```python
from build123d import *

# Parameters (mm, degrees)
F1_DEPTH = 50
F2_DEPTH = 25


with BuildPart() as f1:
    # F0 (on Front) → F1 (new body)
    with BuildSketch(Plane.XZ):
        with BuildLine():
            ThreePointArc((60.3004275437, 340.9588258691), (82.833452945, 336.1958976151), (105, 329.9455447494))
            Line((105, 329.9455447494), (105, 360))
            ThreePointArc((105, 360), (0, 375), (-105, 360))
            Line((-105, 360), (-105, 329.9455447494))
            ThreePointArc((-105, 329.9455447494), (-82.833452945, 336.1958976151), (-60.3004275437, 340.9588258691))
            ThreePointArc((-60.3004275437, 340.9588258691), (-44.7093862816, 361.4956891559), (-24.5847162741, 345.3761054643))
            ThreePointArc((-24.5847162741, 345.3761054643), (-17.7950983093, 345.7924189108), (-10.9986121712, 346.0752707581))
            ThreePointArc((-10.9986121712, 346.0752707581), (-0.0873673767, 357.2496530373), (11, 346.25))
            ThreePointArc((11, 346.25), (10.9996530373, 346.1626326233), (10.9986121712, 346.0752707581))
            ThreePointArc((10.9986121712, 346.0752707581), (17.7950983093, 345.7924189108), (24.5847162741, 345.3761054643))
            ThreePointArc((24.5847162741, 345.3761054643), (43.3731818064, 361.6106063163), (60.5, 343.6317978593))
            ThreePointArc((60.5, 343.6317978593), (60.4500375457, 342.2915918653), (60.3004275437, 340.9588258691))
        make_face()
        with BuildLine():
            ThreePointArc((-105, 299.635194862), (0, 317.5), (105, 299.635194862))
            Line((105, 299.635194862), (105, 329.9455447494))
            ThreePointArc((105, 329.9455447494), (82.833452945, 336.1958976151), (60.3004275437, 340.9588258691))
            ThreePointArc((60.3004275437, 340.9588258691), (40.2906137184, 325.7679065626), (24.5847162741, 345.3761054643))
            ThreePointArc((24.5847162741, 345.3761054643), (17.7950983093, 345.7924189108), (10.9986121712, 346.0752707581))
            ThreePointArc((10.9986121712, 346.0752707581), (0, 335.25), (-10.9986121712, 346.0752707581))
            ThreePointArc((-10.9986121712, 346.0752707581), (-17.7950983093, 345.7924189108), (-24.5847162741, 345.3761054643))
            ThreePointArc((-24.5847162741, 345.3761054643), (-24.521191543, 344.5049796657), (-24.5, 343.6317978593))
            ThreePointArc((-24.5, 343.6317978593), (-41.159794006, 325.6817603135), (-60.3004275437, 340.9588258691))
            ThreePointArc((-60.3004275437, 340.9588258691), (-82.833452945, 336.1958976151), (-105, 329.9455447494))
            Line((-105, 329.9455447494), (-105, 299.635194862))
        make_face()
        with BuildLine():
            ThreePointArc((-24.5847162741, 345.3761054643), (-44.7093862816, 361.4956891559), (-60.3004275437, 340.9588258691))
            ThreePointArc((-60.3004275437, 340.9588258691), (-57.8364575566, 341.3854224733), (-55.3694709553, 341.7942132133))
            ThreePointArc((-55.3694709553, 341.7942132133), (-44.09566787, 356.5334971291), (-29.5706194929, 344.9849865759))
            ThreePointArc((-29.5706194929, 344.9849865759), (-27.0783740558, 345.1895481594), (-24.5847162741, 345.3761054643))
        make_face()
        with BuildLine():
            ThreePointArc((-55.3694709553, 341.7942132133), (-57.8364575566, 341.3854224733), (-60.3004275437, 340.9588258691))
            ThreePointArc((-60.3004275437, 340.9588258691), (-41.159794006, 325.6817603135), (-24.5, 343.6317978593))
            ThreePointArc((-24.5, 343.6317978593), (-24.521191543, 344.5049796657), (-24.5847162741, 345.3761054643))
            ThreePointArc((-24.5847162741, 345.3761054643), (-27.0783740558, 345.1895481594), (-29.5706194929, 344.9849865759))
            ThreePointArc((-29.5706194929, 344.9849865759), (-29.5176668778, 344.3093129543), (-29.5, 343.6317978593))
            ThreePointArc((-29.5, 343.6317978593), (-41.5788926281, 330.6644711799), (-55.3694709553, 341.7942132133))
        make_face()
        with BuildLine():
            ThreePointArc((55.3694709553, 341.7942132133), (57.8364575566, 341.3854224733), (60.3004275437, 340.9588258691))
            ThreePointArc((60.3004275437, 340.9588258691), (60.4500375457, 342.2915918653), (60.5, 343.6317978593))
            ThreePointArc((60.5, 343.6317978593), (43.3731818064, 361.6106063163), (24.5847162741, 345.3761054643))
            ThreePointArc((24.5847162741, 345.3761054643), (27.0783740558, 345.1895481594), (29.5706194929, 344.9849865759))
            ThreePointArc((29.5706194929, 344.9849865759), (43.177515095, 356.6141309815), (55.5, 343.6317978593))
            ThreePointArc((55.5, 343.6317978593), (55.4673266794, 342.7106904874), (55.3694709553, 341.7942132133))
        make_face()
        with BuildLine():
            ThreePointArc((24.5847162741, 345.3761054643), (40.2906137184, 325.7679065626), (60.3004275437, 340.9588258691))
            ThreePointArc((60.3004275437, 340.9588258691), (57.8364575566, 341.3854224733), (55.3694709553, 341.7942132133))
            ThreePointArc((55.3694709553, 341.7942132133), (40.90433213, 330.7300985895), (29.5706194929, 344.9849865759))
            ThreePointArc((29.5706194929, 344.9849865759), (27.0783740558, 345.1895481594), (24.5847162741, 345.3761054643))
        make_face()
    extrude(amount=-F1_DEPTH)

    # F0 (on Front) → F2 (cut)
    with BuildSketch(Plane.XZ):
        with BuildLine():
            ThreePointArc((-24.5847162741, 345.3761054643), (-44.7093862816, 361.4956891559), (-60.3004275437, 340.9588258691))
            ThreePointArc((-60.3004275437, 340.9588258691), (-57.8364575566, 341.3854224733), (-55.3694709553, 341.7942132133))
            ThreePointArc((-55.3694709553, 341.7942132133), (-44.09566787, 356.5334971291), (-29.5706194929, 344.9849865759))
            ThreePointArc((-29.5706194929, 344.9849865759), (-27.0783740558, 345.1895481594), (-24.5847162741, 345.3761054643))
        make_face()
        with BuildLine():
            ThreePointArc((-55.3694709553, 341.7942132133), (-57.8364575566, 341.3854224733), (-60.3004275437, 340.9588258691))
            ThreePointArc((-60.3004275437, 340.9588258691), (-41.159794006, 325.6817603135), (-24.5, 343.6317978593))
            ThreePointArc((-24.5, 343.6317978593), (-24.521191543, 344.5049796657), (-24.5847162741, 345.3761054643))
            ThreePointArc((-24.5847162741, 345.3761054643), (-27.0783740558, 345.1895481594), (-29.5706194929, 344.9849865759))
            ThreePointArc((-29.5706194929, 344.9849865759), (-29.5176668778, 344.3093129543), (-29.5, 343.6317978593))
            ThreePointArc((-29.5, 343.6317978593), (-41.5788926281, 330.6644711799), (-55.3694709553, 341.7942132133))
        make_face()
        with BuildLine():
            ThreePointArc((55.3694709553, 341.7942132133), (57.8364575566, 341.3854224733), (60.3004275437, 340.9588258691))
            ThreePointArc((60.3004275437, 340.9588258691), (60.4500375457, 342.2915918653), (60.5, 343.6317978593))
            ThreePointArc((60.5, 343.6317978593), (43.3731818064, 361.6106063163), (24.5847162741, 345.3761054643))
            ThreePointArc((24.5847162741, 345.3761054643), (27.0783740558, 345.1895481594), (29.5706194929, 344.9849865759))
            ThreePointArc((29.5706194929, 344.9849865759), (43.177515095, 356.6141309815), (55.5, 343.6317978593))
            ThreePointArc((55.5, 343.6317978593), (55.4673266794, 342.7106904874), (55.3694709553, 341.7942132133))
        make_face()
        with BuildLine():
            ThreePointArc((24.5847162741, 345.3761054643), (40.2906137184, 325.7679065626), (60.3004275437, 340.9588258691))
            ThreePointArc((60.3004275437, 340.9588258691), (57.8364575566, 341.3854224733), (55.3694709553, 341.7942132133))
            ThreePointArc((55.3694709553, 341.7942132133), (40.90433213, 330.7300985895), (29.5706194929, 344.9849865759))
            ThreePointArc((29.5706194929, 344.9849865759), (27.0783740558, 345.1895481594), (24.5847162741, 345.3761054643))
        make_face()
    extrude(amount=-F2_DEPTH, mode=Mode.SUBTRACT)


solid = f1.part
```
Verification items for the finished model (mm, model axes). A direction names the side the tool comes from. Give positions to 0.01 mm unless a question says otherwise; leave off trailing zeros. Loops run counter-clockwise (first coordinate to the right, second up) from the corner with the lowest first, then second, coordinate; pieces in that order, holes last.
1. Section check B-B, the plane x = 0. Enter the section's corners in (y, z).
2. Mould release check, pull along X, two halves, no side actions. Record for faces 3 (the cylindrical face through (-1.498, 24.65, 317.496)), 4 (the flat face through (105, 25, 329)), 5 (the flat face through (-1, 0, 329)): released by +X, released by -X, zero draft, split by the parting line, or undercut.
3. Go/stop test with flat-tipped pins: pin 1 Ø8 at (x, y) = (33, 23.5) entering from -Z; pin 2 Ø12 at (x, y) = (16, 28.5) entering from -Z; pin 3 Ø11 at (x, z) = (46, 352.5) entering from -Y. Record where each tip stops, or that it passes through.
4. Thickness scan on line 1 (X direction, y = 32, z = 347); line 2 (X direction, y = 5.5, z = 355); line 3 (Z direction, x = -54.5, y = 24). Record the ranges inside material, lowest first.
5. Set-up check for faces 1 (the flat face through (52, 25, 353)), 2 (the cylindrical face through (1, 25, 375)): record each of +Z, -Z, +X, -X, +Y, -Y from which the full face is reachable in a straight line by a thin tool's end or side.
6. Section check D-D, the plane x = 42.5. Enter the section's corners in (y, z), then the cut area to 3 significant figures.
7. Section check A-A, the plane y = 29. Enter the section's corners in (x, z).
8. Section check C-C, the plane z = 314. Enter the section's corners in (x, y), then the cut area to 3 significant figures.
Geometry says:
1. outline: (0, 317.5) - (50, 317.5) - (50, 335.25) - (0, 335.25) - close; (0, 357.25) - (50, 357.25) - (50, 375) - (0, 375) - close
2. face 3: undercut
2. face 4: released by +X
2. face 5: zero draft
3. pin 1: stops at z = 315.34
3. pin 2: stops at z = 316.74
3. pin 3: stops at y = 25
4. line 1: x = -105 to -55.06, -29.94 to -10.97, 10.97 to 29.94, 55.06 to 105
4. line 2: x = -105 to -56.46, -28.54 to -6.67, 6.67 to 28.54, 56.46 to 105
4. line 3: z = 312.79 to 330.22, 357.05 to 371.02
5. face 1: -Y
5. face 2: +Z, +Y, -Y
6. outline: (0, 314.64) - (50, 314.64) - (50, 330.63) - (25, 330.63) - (25, 325.63) - (0, 325.63) - close; (0, 361.63) - (25, 361.63) - (25, 356.63) - (50, 356.63) - (50, 372.58) - (0, 372.58) - close
6. area: 1,350 mm2
7. outline: (-105, 299.64) arc R317.5 cw to (105, 299.64) - (105, 360) arc R375 ccw to (-105, 360) - close; hole circle Ø26 at (-42.5, 343.63); hole (11, 346.08) arc R11 ccw to (11, 346.25) arc R11 ccw (long way) to start; hole circle Ø26 at (42.5, 343.63)
8. outline: (-105, 0) - (-47.01, 0) - (-47.01, 50) - (-105, 50) - close; (47.01, 0) - (105, 0) - (105, 50) - (47.01, 50) - close
8. area: 5,800 mm2
